Autodesk Inventor part; units mm, degrees
ref_plane "YZ Plane" through (0, 0, 0) normal (1, 0, 0) x (0, 1, 0)
ref_plane "XZ Plane" through (0, 0, 0) normal (0, 1, 0) x (-1, 0, 0)
ref_plane "XY Plane" through (0, 0, 0) normal (0, 0, 1) x (1, 0, 0)
sketch "Sketch1" plane through (0, 0, 0) normal (0, 0, 1) x (1, 0, 0)
  line L0 (0, 0) -> (-89.8017, 0) construction
  line L1 (-89.8017, 0) -> (-44.90085, 44.901711) construction
  line L2 (-44.90085, 44.901711) -> (0, 0) construction
  arc A0 (-44.196, 0) -> (0.000848, 44.196) centre (0, 0) ccw
  line L3 (-44.196, 0) -> (-44.196, 44.196848) construction
  line L4 (-44.196, 44.196848) -> (-44.90085, 44.901711) construction
  circle A1 centre (-44.90085, 44.901711) radius 5.715
  arc A2 (-44.196, 0) -> (0.000848, 44.196) centre (-44.196, 44.196848) ccw
  dimension "d8" = 89.8017
  dimension "d9" = 63.5
  dimension "d10" = 63.5
  dimension "d11" = 44.196
  dimension "d12" = 11.43
extrude "Extrusion1" add sketch "Sketch1" along normal blind 13.97 and the other way blind 1.27
sketch "Sketch5" plane through (0, 0, 13.97) normal (0, 0, 1) x (1, 0, 0)
  line L0 (2.846729, 10.62373) -> (7.777055, -7.777205)
  line L1 (7.777055, -7.777205) -> (-10.623784, -2.846525)
  line L2 (-10.623784, -2.846525) -> (2.846729, 10.62373)
  line L3 (0, 0) -> (-12.944409, 12.944657) construction
  arc A0 (-44.196, 0) -> (0.000848, 44.196) centre (-44.196, 44.196848) ccw
  dimension "d31" = 19.05
extrude "Extrusion4" cut sketch "Sketch5" against normal through all
sketch "Sketch6" plane through (0, 0, -1.27) normal (0, 0, -1) x (-1, 0, 0)
  circle A0 centre (0, 0) radius 6.35
  dimension "d34" = 12.7
extrude "Extrusion5" add sketch "Sketch6" along normal blind 8.466667 and the other way blind 21.166667
sketch "Sketch7" plane through (0, 0, 13.97) normal (0, 0, 1) x (1, 0, 0)
  circle A0 centre (0, 0) radius 12.7
  dimension "d39" = 25.4
extrude "Extrusion6" add sketch "Sketch7" against normal up to surface (15.24 mm away)
sketch "Sketch8" plane through (0, 0, -9.736667) normal (0, 0, -1) x (-1, 0, 0)
  circle A0 centre (0, 0) radius 6.35
  line L0 (4.490085, 4.490171) -> (1.64356, -6.133613)
  line L1 (1.64356, -6.133613) -> (-6.133645, 1.643442)
  line L2 (-6.133645, 1.643442) -> (4.490085, 4.490171)
  circle A1 centre (44.90085, 44.901711) radius 5.715
  line L3 (44.90085, 44.901711) -> (0, 0)
extrude "Extrusion7" add sketch "Sketch8" along normal blind 12.7 contours L0 L1 L2
ref_plane "Work Plane1" through (-44.90085, 44.901711, 7.196667) normal (0, 0, -1) x (-1, 0, 0)
sketch "Sketch9" plane through (0, 0, 19.896667) normal (0, 0, 1) x (1, 0, 0)
  circle A0 centre (0, 0) radius 6.35
extrude "Extrusion8" add sketch "Sketch9" along normal blind 1.27
sketch "Sketch10" plane through (0, 0, 13.97) normal (0, 0, 1) x (1, 0, 0)
  circle A0 centre (0, 0) radius 6.35
extrude "Extrusion9" add sketch "Sketch10" along normal blind 8.466667
sketch "Sketch11" plane through (0, 0, 13.97) normal (0, 0, 1) x (1, 0, 0)
  circle A0 centre (0, 0) radius 8.466667
  circle A1 centre (0, 0) radius 10.16
  arc A2 (-44.196, 0) -> (0.000848, 44.196) centre (-44.196, 44.196848) ccw
  arc A3 (-22.076558, 5.933398) -> (-5.932974, 22.076671) centre (0, 0) ccw
  arc A4 (-24.069883, 4.848395) -> (-4.847933, 24.069976) centre (0, 0) ccw
  arc A5 (-44.196, 0) -> (0.000848, 44.196) centre (0, 0) ccw
  circle A6 centre (0, 0) radius 50.8
  point P0 (-37.249283, 0.549345)
  point P1 (-0.548631, 37.249293)
  point P2 (-38.945409, 0.312994)
  point P3 (-0.312247, 38.945415)
  dimension "d51" = 16.93333
  dimension "d52" = 1.69333
  dimension "d53" = 1.69333
  dimension "d55" = 12.7
  dimension "d61" = 101.6
sketch "Sketch11 outline for Extrusion10" plane through (0, 0, 13.97) normal (0, 0, 1) x (1, 0, 0)
  circle A0 centre (0, 0) radius 50.8
  circle A1 centre (0, 0) radius 10.16
  arc A2 (-5.932974, 22.076671) -> (-22.076558, 5.933398) centre (0, 0) cw
  arc A3 (-22.076558, 5.933398) -> (-24.069883, 4.848395) centre (-44.196, 44.196848) cw
  arc A4 (-24.069883, 4.848395) -> (-4.847933, 24.069976) centre (0, 0) ccw
  arc A5 (-4.847933, 24.069976) -> (-5.932974, 22.076671) centre (-44.196, 44.196848) cw
  circle A6 centre (0, 0) radius 8.466667
extrude "Extrusion10" cut sketch "Sketch11 outline for Extrusion10" against normal blind 1.27 draft -10
sketch "Sketch12" plane through (0, 0, 22.436667) normal (0, 0, 1) x (1, 0, 0)
  circle A0 centre (0, 0) radius 6.35
extrude "Extrusion11" add sketch "Sketch12" against normal up to surface (9.736667 mm away)
ref_plane "Work Plane2" through (0, 0, 6.35) normal (0, 0, 1) x (1, 0, 0)
mirror "Mirror1" about plane through (0, 0, 6.35) normal (0, 0, 1) of "Extrusion10"
sketch "Sketch14" plane through (-44.90085, 44.901711, -1.27) normal (0, 0, -1) x (-1, 0, 0)
  circle A0 centre (0, 0) radius 5.715
  point P0 (-44.90085, -44.901711)
extrude "Extrusion12" cut sketch "Sketch14" against normal blind 1.27
sketch "Sketch15" plane through (-44.90085, 44.901711, 13.97) normal (0, 0, 1) x (1, 0, 0)
  circle A0 centre (0, 0) radius 5.715
  point P0 (44.90085, -44.901711)
extrude "Extrusion13" cut sketch "Sketch15" against normal blind 1.27
ref_plane "Work Plane3" through (-12.944409, 12.944657, 0) normal (-0.7071136, -0.7071, 0) x (0.7071, -0.7071136, 0)
sketch "Sketch17" plane through (-12.944409, 12.944657, 0) normal (-0.7071136, -0.7071, 0) x (0.7071, -0.7071136, 0)
  line L0 (-50.908666, 12.7) -> (-39.478666, 12.7)
  line L1 (-39.478666, 12.7) -> (0, 12.7)
  line L2 (0, 12.7) -> (0, 9.313333)
  line L3 (0, 9.313333) -> (-39.478666, 9.313333)
  line L4 (-39.478666, 9.313333) -> (-39.478666, 12.7)
  line L5 (0, 12.7) -> (0, 0)
  line L6 (-39.478666, 12.7) -> (-45.193666, 12.7)
  line L7 (-45.193666, 12.7) -> (-45.193666, 9.313333)
  line L8 (-45.193666, 9.313333) -> (-39.478666, 9.313333)
  line L9 (-39.478666, 9.313333) -> (-39.478666, 12.7)
  line L10 (-39.478666, 0) -> (-50.908666, 0)
  point P0 (18.306334, 0)
  point P1 (-45.193666, 0)
  dimension "d69" = 3.38667
extrude "Extrusion14" add sketch "Sketch17" along normal mid plane 11.43
sketch "Sketch18" plane through (0, 0, -22.436667) normal (0, 0, -1) x (-1, 0, 0)
  circle A0 centre (0, 0) radius 6.35
  dimension "d72" = 12.7
extrude "Extrusion15" cut sketch "Sketch18" against normal through all
sketch "Sketch19" plane through (0, 0, 0) normal (0, 0, -1) x (-1, 0, 0)
  circle A0 centre (0, 0) radius 6.35
  line L0 (6.35, 0.000061) -> (0.000061, -6.35)
  line L1 (0.000061, -6.35) -> (-6.35, -0.000061)
  line L2 (-6.35, -0.000061) -> (-0.000061, 6.35)
  line L3 (-0.000061, 6.35) -> (6.35, 0.000061)
  circle A1 centre (44.90085, 44.901711) radius 5.715 construction
  line L4 (44.90085, 44.901711) -> (0, 0) construction
extrude "Extrusion16" add sketch "Sketch19" against normal up to surface (12.7 mm away) contours L3 A0 | A0 L0 | L2 A0 | A0 L1
properties part number "Geneva Drive" material "ABS Plastic"
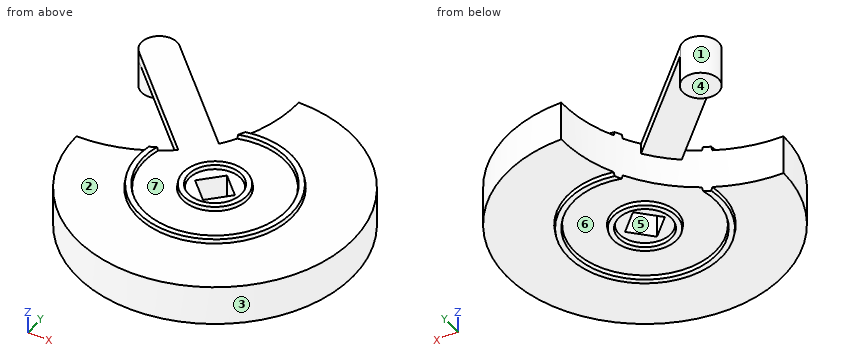
Can you work these out from the model? Positions are in its coordinate system, mm. Face numbers are marked on the shaded views. A direction names the side the tool comes from. Coordinates: 2 decimals unless noted, no trailing zeros. Write each loop counter-clockwise with the first axis right and the second up, starting at its lowest first coordinate (ties: lowest second). Pieces come first, ordered by that corner, then holes. Notation, with made-up numbers: (17, 36) - (51, 36) arc R19 ccw to (51, 47) - close; hole circle Ø6 at (81.25, -8.5). An arc over 180 degrees is marked (long way). Return JSON: item names as keys, results as strings.
Q1. If we section it at C-C (x = 38): Please give me the cut outline in (y, z), then the cut area to 3 significant figures.
Computed values:
{"outline": "(-22.57, 0) - (22.57, 0) - (22.57, 12.7) - (-22.57, 12.7) - close", "area": "573 mm2"}
Q2. On a 3-axis mill with a long thin cutter (end or side, diameter ignored), from which of +Z, -Z, +X, -X, +Y, -Y can I reach the whole of each face in a straight line? I mean the marked faces 4, 5, 6 and 7. Say none if no direction works.
Computed values:
{"face 4": "-Z, +X, -X, +Y, -Y", "face 5": "+Z, -Z", "face 6": "-Z", "face 7": "+Z"}
Q3. If we section it at D-D (y = -27): Please give me the cut outline in (x, z).
Computed values:
{"outline": "(-34.99, 0) - (34.99, 0) - (34.99, 12.7) - (-34.99, 12.7) - close"}
Q4. I'm going to push flat-ended pins straight in: pin 1 Ø3 at (x, z) = (-18, 4) entering from -Y; pin 2 Ø6 at (x, z) = (-38, 9.5) entering from -Y; pin 3 Ø1.5 at (x, z) = (-16.5, 11) entering from -Y. Where does each tip first touch, or does it pass through?
Computed values:
{"pin 1": "stops at y = -41", "pin 2": "stops at y = -26.99", "pin 3": "stops at y = -41.29"}
Q5. Thinking about a two-plate mould opening in Y: for the marked faces 1, 2 and 3, which applies, +Y half, -Y half, draft (parallel to the pull), parting line (faces both ways), or undercut?
Computed values:
{"face 1": "undercut", "face 2": "draft", "face 3": "parting line"}
Q6. Please list where these lines run through material, in increasing order: L1, parallel to Z at x = 13, y = -39.5; L2, parallel to X at y = 4, z = 2; L3, parallel to X at y = 31, z = 10.5. Write a range as from..to.
Computed values:
{"L1": "z = 0..12.7", "L2": "x = -25.82..-2.35, 2.35..44.01", "L3": "x = -39.08..-22.92, -2.02..31.5"}
Q7. If we section it at A-A (z = 5.25): Please give me the cut outline in (x, y) (3 decimals), then the cut area to 3 significant figures.
Computed values:
{"outline": "circle Ø11.43 at (-44.901, 44.902); (-44.196, 0) arc R44.196 ccw (long way) to (0.001, 44.196) arc R44.197 cw to start; hole (-6.35, 0) - (0, -6.35) - (6.35, 0) - (0, 6.35) - close", "area": "5,040 mm2"}
